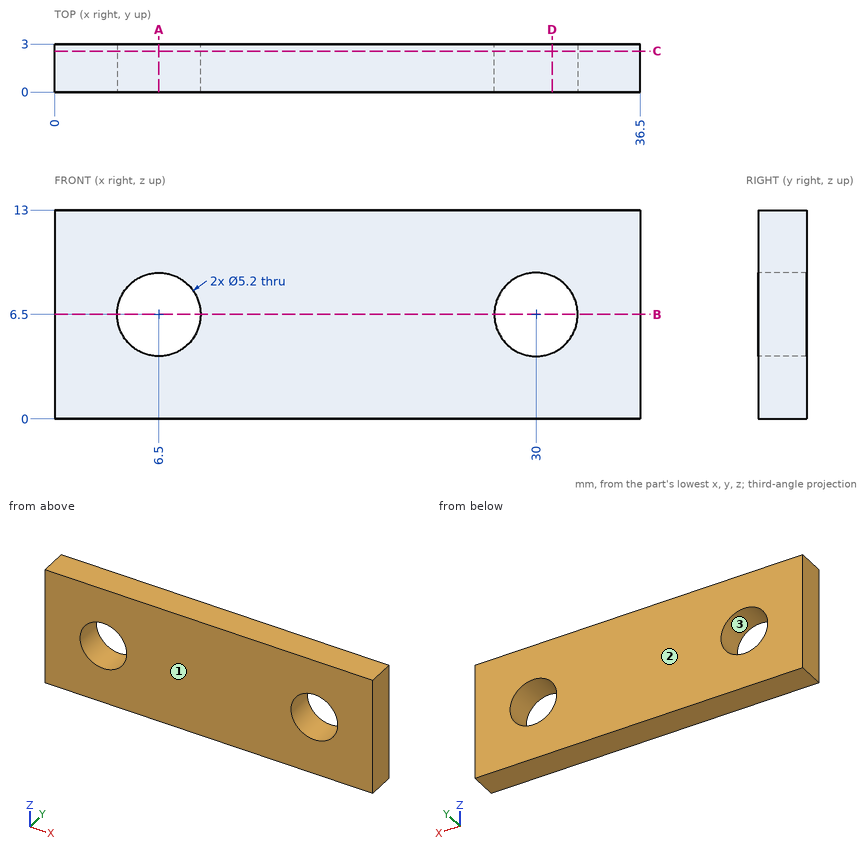
Job drawing, mm, ordinate dimensions from the low corner. One solid piece. Give positions to 0.01 mm unless a question says otherwise; leave off trailing zeros. Loops run counter-clockwise (first coordinate to the right, second up) from the corner with the lowest first, then second, coordinate; pieces in that order, holes last. Notation, with made-up numbers: (-29.75, 51) -> (20.25, 51) arc R15 ccw to (20.25, 74) -> close; hole circle Ø1 at (75.5, 80). An arc over 180 degrees is marked (long way). Use a Markdown table: item, result. Add a question column.
(1) Wall check: line 1 along X through (y, z) = (1.7, 6.5); line 2 along X through (y, z) = (1.4, 5.25); line 3 along Z through (x, y) = (30, 1.3). Give the ranges that are in metal, low to high.
(2) Slice it at D-D on x = 31. List the corners of the cut face in (y, z), and give its area (3 significant figures).
(3) Slice it at C-C on y = 2.55. List the corners of the cut face in (x, z), and give its area (3 significant figures).
(4) Slice it at B-B on z = 6.5. List the corners of the cut face in (x, y), and give its area (3 significant figures).
(5) Mould opens along Y. For the marked faces 1, 2 and 3 say: +Y half, -Y half, draft (parallel to the pull), parting line (faces both ways), or undercut.
(6) Slice it at A-A on x = 6.5. List the corners of the cut face in (y, z).
Filled sheet:
| question | item | result |
|---|---|---|
| 1 | line 1 | 0 to 3.9, 9.1 to 27.4, 32.6 to 36.5 |
| 1 | line 2 | 0 to 4.22, 8.78 to 27.72, 32.28 to 36.5 |
| 1 | line 3 | 0 to 3.9, 9.1 to 13 |
| 2 | outline | (0, 0) -> (3, 0) -> (3, 4.1) -> (0, 4.1) -> close; (0, 8.9) -> (3, 8.9) -> (3, 13) -> (0, 13) -> close |
| 2 | area | 24.6 mm2 |
| 3 | outline | (0, 0) -> (36.5, 0) -> (36.5, 13) -> (0, 13) -> close; hole circle Ø5.2 at (6.5, 6.5); hole circle Ø5.2 at (30, 6.5) |
| 3 | area | 432 mm2 |
| 4 | outline | (0, 0) -> (3.9, 0) -> (3.9, 3) -> (0, 3) -> close; (9.1, 0) -> (27.4, 0) -> (27.4, 3) -> (9.1, 3) -> close; (32.6, 0) -> (36.5, 0) -> (36.5, 3) -> (32.6, 3) -> close |
| 4 | area | 78.3 mm2 |
| 5 | face 1 | -Y half |
| 5 | face 2 | +Y half |
| 5 | face 3 | draft |
| 6 | outline | (0, 0) -> (3, 0) -> (3, 3.9) -> (0, 3.9) -> close; (0, 9.1) -> (3, 9.1) -> (3, 13) -> (0, 13) -> close |
